Here's how the part is built. I have some questions about the finished solid (model axes, mm). Face numbers are marked on the shaded views. A direction names the side the tool comes from. Coordinates: 2 decimals unless noted, no trailing zeros. Loops run counter-clockwise (first coordinate to the right, second up) from the corner with the lowest first, then second, coordinate; pieces in that order, holes last. Notation, with made-up numbers: (50.5, 48.25) -> (55.5, 48.25) arc R26 ccw to (55.5, 76.25) -> close; hole circle Ø4 at (38, -12.5). An arc over 180 degrees is marked (long way). Use CSV: the item, a comma, the result in double quotes. Start each with the question number.
from build123d import *

# Parameters (mm, degrees)
F3_DEPTH = 25
F4_DEPTH = 25


with BuildPart() as f1:
    # F0 (on Front) → F1 (revolve)
    with BuildSketch(Plane.XZ):
        Polygon((0, 27.977053), (0, -22.563635), (16.162515, -22.563635), (15.007145, -19.202555), (12.906471, -19.202555), (10.490696, -14.476041), (9.020226, -8.48912), (9.020226, -3.762604), (12.596551, 9.510701), (13.896568, 15.825069), (9.020226, 16.829022), (9.020226, 28.639521), (4.610734, 26.410921), (4.610734, 36.439623), (9.813699, 44.771921), (6.656515, 51.64344), (3.127897, 48.393397), (0, 56.936365), (0, 47.673344), (0, 47.410701), (0, 32.768778), align=None)
    revolve(axis=Axis((0, 0, 42.456709), (0, 0, -1)))

    # F2 (on Front) → F3 (cut)
    with BuildSketch(Plane.XZ):
        Polygon((-4.498249, 48.772931), (-8.376098, 51.58437), (-9.137458, 50.469015), (-5.290595, 47.68004), align=None)
    extrude(amount=-F3_DEPTH, mode=Mode.SUBTRACT)

    # F2 (on Front) → F4 (cut)
    with BuildSketch(Plane.XZ):
        Polygon((-4.498249, 48.772931), (-8.376098, 51.58437), (-9.137458, 50.469015), (-5.290595, 47.68004), align=None)
    extrude(amount=F4_DEPTH, mode=Mode.SUBTRACT)


solid = f1.part
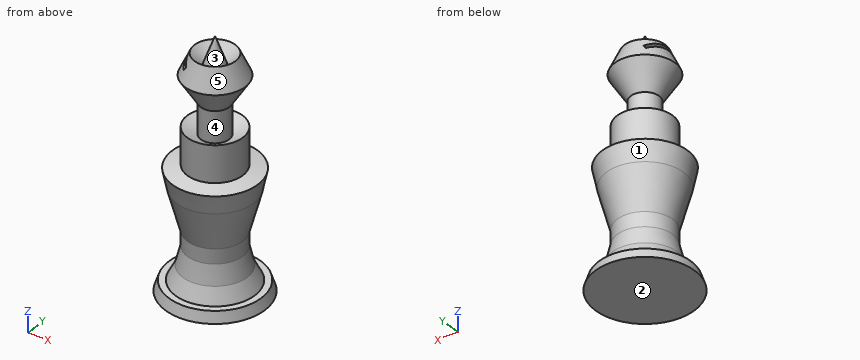
1) Please list where these lines run through material, in increasing order: L1, parallel to Z at x = 4, y = -4.5; L2, parallel to Z at x = -6.5, y = -3; L3, parallel to Z at x = 2, y = -14.5. Write a range as [from, to].
2) For P1, Ø12, axis at x = -6.5, y = 8.5, coming from the +Z side; P2, Ø3, axis at y = 3, z = 26, coming from the -X side; P3, Ø3, axis at x = 4, z = -6.5, coming from the +Y side, each with a flat end and sliding along its axis, tell me the tip position at first contact or that it passes through.
3) Which directions (+Z, -Z, +X, -X, +Y, -Y) give clear straight access to the entire face, cutting with the end or side of a thin tool? Please do the marked faces 4 and 5.
4) I want a section at A-A, the plane z = -2. Please give me the cut outline in (x, y), plus the area to 3 significant figures.
5) Thinking about a two-plate mould opening in X: for the marked faces 1, 2 and 3, which applies, pulls with the +X half, pulls with the -X half, needs draft (parallel to the pull), parting line crosses it, or undercut?
Return value:
1,L1,"z = [-22.56, 27.12], [38.7, 51.06]"
1,L2,"z = [-22.56, 27.7], [40.52, 48.56], [50.22, 50.55]"
1,L3,"z = [-22.56, -19.2]"
2,P1,"stops at z = 51.64"
2,P2,"stops at x = -8.89"
2,P3,"stops at y = 8.67"
3,face 4,"none"
3,face 5,"+Z"
4,outline,"circle Ø18.99 at (0, 0)"
4,area,"283 mm²"
5,face 1,"parting line crosses it"
5,face 2,"needs draft"
5,face 3,"undercut"
